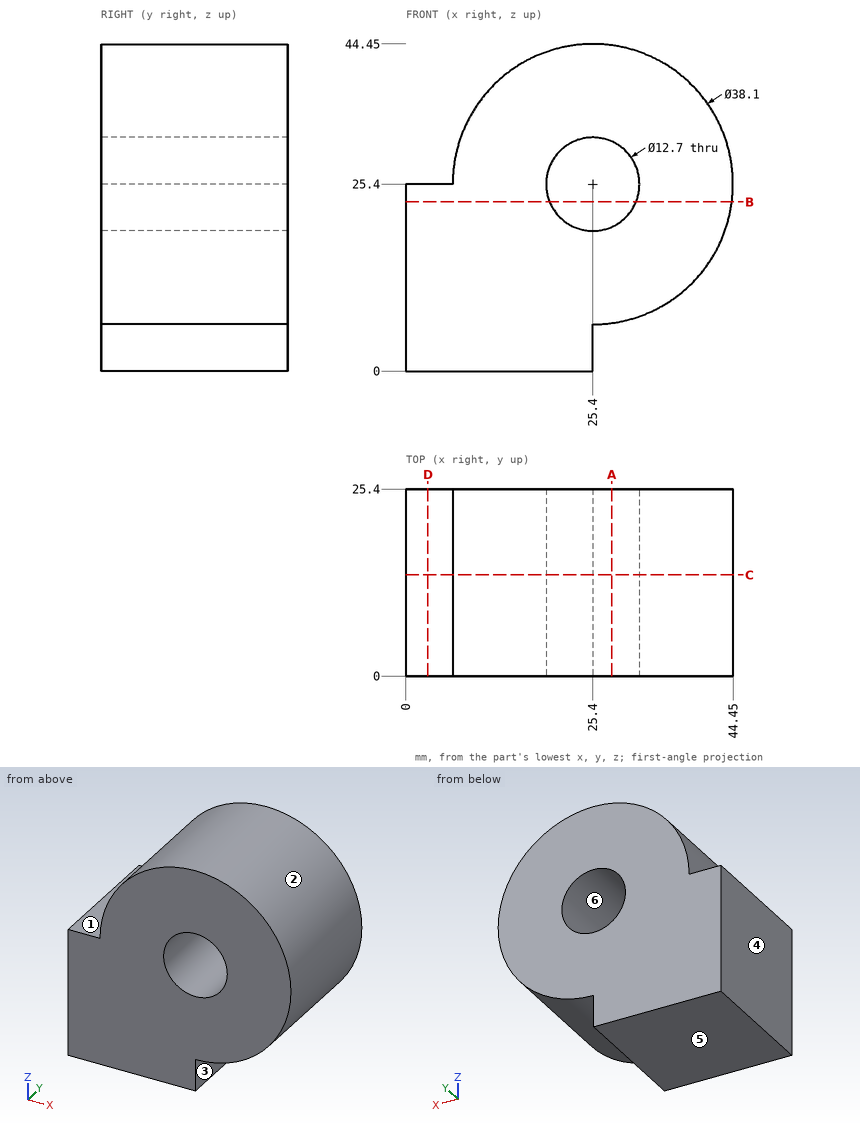
Part print with two shaded views. Sizes in mm from the minimum x, y, z corner. A direction names the side the tool comes from. Round coordinates to 2 decimals unless told otherwise and drop trailing zeros. Write each loop counter-clockwise with the first axis right and the second up, starting at its lowest first coordinate (ties: lowest second). Pieces come first, ordered by that corner, then holes. Notation, with made-up numbers: (52, 42.25) - (83, 42.25) arc R14 cw to (83, 65.25) - close; hole circle Ø9 at (49, 73.25). An arc over 180 degrees is marked (long way). Answer as CSV lines item,"result".
Q1. Cut at D-D (x = 3). Write the cut outline in (y, z).
Report:
outline,"(0, 0) - (25.4, 0) - (25.4, 25.4) - (0, 25.4) - close"
Q2. Pull direction X, two halves, no side cores. Call the marked faces 4, 5 and 6: +X half, -X half, draft (parallel to the pull), parting line (faces both ways), or undercut.
Report:
face 4,"-X half"
face 5,"draft"
face 6,"undercut"
Q3. Drill centre lines: probe 1 along Z at (x, y) = (25, 12.75); probe 2 along X at (y, z) = (6.5, 6); probe 3 along Z at (x, y) = (30.5, 13.5). Where is each one in solid material? Low to high. Write a range as [from, to].
Report:
probe 1,"z = [0, 19.06], [31.74, 44.45]"
probe 2,"x = [0, 25.4]"
probe 3,"z = [7.05, 21.62], [29.18, 43.75]"
Q4. Cut at C-C (y = 13.75). Write the cut outline in (x, z), and give its area (3 significant figures).
Report:
outline,"(0, 0) - (25.4, 0) - (25.4, 6.35) arc R19.05 ccw (long way) to (6.35, 25.4) - (0, 25.4) - close; hole circle Ø12.7 at (25.4, 25.4)"
area,"1,370 mm^2"
Q5. Cut at B-B (z = 23). Write the cut outline in (x, y).
Report:
outline,"(0, 0) - (19.52, 0) - (19.52, 25.4) - (0, 25.4) - close; (31.28, 0) - (44.3, 0) - (44.3, 25.4) - (31.28, 25.4) - close"
Q6. Cut at A-A (x = 28). Write the cut outline in (y, z), and give its area (3 significant figures).
Report:
outline,"(0, 6.53) - (25.4, 6.53) - (25.4, 19.61) - (0, 19.61) - close; (0, 31.19) - (25.4, 31.19) - (25.4, 44.27) - (0, 44.27) - close"
area,"664 mm^2"
Q7. Tool access for the marked faces 1, 2 and 3: list every direction of +Z, -Z, +X, -X, +Y, -Y with a clear straight run to the whole face (end or side of a thin tool).
Report:
face 1,"+Z, -X, +Y, -Y"
face 2,"+Y, -Y"
face 3,"-Z, +X, +Y, -Y"
Q8. Drop flat-ended pins along their axis: pin 1 (8 mm diameter, centred on y = 8.5, z = 14.5, fed in from +X); pin 2 (3 mm diameter, centred on x = 31.5, y = 9.5, fed in from -Z); pin 3 (4 mm diameter, centred on x = 8, y = 15.5, fed in from +Z). Give the stop position or say it passes through.
Report:
pin 1,"stops at x = 43.16"
pin 2,"stops at z = 6.91"
pin 3,"stops at z = 36.61"
